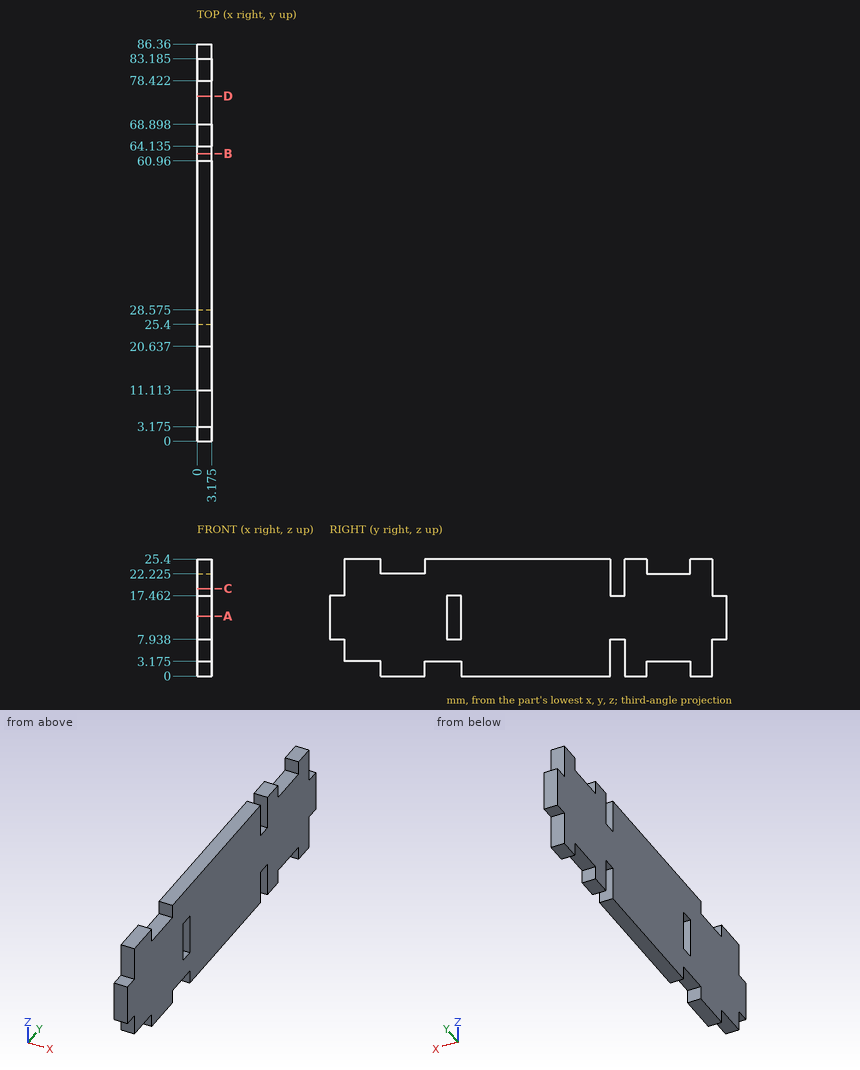
The drawing under review shows one solid part. Ordinate dimensions are in mm from its lowest x, y, z. Give positions to 0.01 mm unless a question says otherwise; leave off trailing zeros. Write each loop counter-clockwise with the first axis right and the second up, starting at its lowest first coordinate (ties: lowest second). Pieces come first, ordered by that corner, then holes. Notation, with made-up numbers: (-5.5, 84) -> (46.5, 84) arc R20 cw to (46.5, 111) -> close; hole circle Ø11 at (-34, -5). An arc over 180 degrees is marked (long way). Answer in a Markdown table with one row per item.
(1) Clearance check with flat-ended pins moving along their axes: pin 1 (1 mm diameter, centred on x = 0.5, y = 25.5, fed in from -Z) (1 decimal); pin 2 (1 mm diameter, centred on x = 1, y = 84.5, fed in from +Z); pin 3 (1.6 mm diameter, centred on x = 2, y = 73, fed in from +Z) (1 decimal). State where each tip first meets the part, or that it passes through.
Results:
| item | result |
|---|---|
| pin 1 | z = 3.2 |
| pin 2 | z = 17.46 |
| pin 3 | z = 22.2 |
(2) Consider section B-B (y = 62.5). State the section outline as (x, z) points (1 decimal).
Results:
| item | result |
|---|---|
| outline | (0, 7.9) -> (3.2, 7.9) -> (3.2, 17.5) -> (0, 17.5) -> close |
(3) To check wall thickness, follow probe 1 along Y at (x, z) = (1.6, 9) (1 decimal); probe 2 along Y at (x, z) = (0.25, 4.5) (1 decimal); probe 3 along Z at (x, y) = (0.7, 27) (1 decimal). State the ranges of each line that lie inside material, in increasing order.
Results:
| item | result |
|---|---|
| probe 1 | 0 to 25.4, 28.6 to 86.4 |
| probe 2 | 3.2 to 61, 64.1 to 83.2 |
| probe 3 | 3.2 to 7.9, 17.5 to 25.4 |
(4) Consider section A-A (z = 13). State the section outline as (x, y) points (1 decimal), then the cut area to 3 significant figures.
Results:
| item | result |
|---|---|
| outline | (0, 0) -> (3.2, 0) -> (3.2, 25.4) -> (0, 25.4) -> close; (0, 28.6) -> (3.2, 28.6) -> (3.2, 86.4) -> (0, 86.4) -> close |
| area | 264 mm2 |
(5) Consider section D-D (y = 75). State the section outline as (x, z) points (1 decimal).
Results:
| item | result |
|---|---|
| outline | (0, 3.2) -> (3.2, 3.2) -> (3.2, 22.2) -> (0, 22.2) -> close |
(6) Consider section C-C (z = 19). State the section outline as (x, y) points (1 decimal), then the cut area to 3 significant figures.
Results:
| item | result |
|---|---|
| outline | (0, 3.2) -> (3.2, 3.2) -> (3.2, 61) -> (0, 61) -> close; (0, 64.1) -> (3.2, 64.1) -> (3.2, 83.2) -> (0, 83.2) -> close |
| area | 244 mm2 |
